from build123d import *

# Parameters (mm, degrees)
SKETCH_1_W          = 25
SKETCH_1_H          = 25
EXTRUDE_1_DEPTH     = 8
SKETCH_2_R          = 1.25
CUT_EXTRUDE_1_DEPTH = 50
SKETCH_3_R          = 1.25
CUT_EXTRUDE_2_DEPTH = 50
CUT_EXTRUDE_4_DEPTH = 10


with BuildPart() as part:
    # Эскиз1 → Бобышка-Вытянуть1 (new body)
    with BuildSketch(Plane.XY):
        Rectangle(SKETCH_1_W, SKETCH_1_H)
    extrude(amount=EXTRUDE_1_DEPTH)

    # Эскиз2 → Вырез-Вытянуть1 (cut)
    with BuildSketch(Plane(origin=(0, 12.5, 0), x_dir=(1, 0, 0), z_dir=(0, 1, 0))):
        with Locations(Location((-7.5, -4, 0), (0, 0, 270))):
            Circle(SKETCH_2_R)
        with Locations(Location((2.5, -4, 0), (0, 0, 270))):
            Circle(SKETCH_2_R)
    extrude(amount=-CUT_EXTRUDE_1_DEPTH, mode=Mode.SUBTRACT)

    # Эскиз3 → Вырез-Вытянуть2 (cut)
    with BuildSketch(Plane(origin=(12.5, 0, 0), x_dir=(0, 0, -1), z_dir=(1, 0, 0))):
        with Locations(Location((-4, 2.5, 0), (0, 0, 90))):
            Circle(SKETCH_3_R)
        with Locations(Location((-4, -7.5, 0), (0, 0, 90))):
            Circle(SKETCH_3_R)
    extrude(amount=-CUT_EXTRUDE_2_DEPTH, mode=Mode.SUBTRACT)

    # Эскиз4 → Вырез-Вытянуть4 (cut)
    with BuildSketch(Plane(origin=(0, 0, 0), x_dir=(-1, 0, 0), z_dir=(0, 0, -1))):
        Polygon((12.5, 7.5), (-7.5, -12.5), (12.5, -12.5), align=None)
    extrude(amount=-CUT_EXTRUDE_4_DEPTH, mode=Mode.SUBTRACT)


solid = part.part
Can you work these out from the model? Positions are in its coordinate system, mm. Give positions to 0.01 mm unless a question says otherwise; leave off trailing zeros. Loops run counter-clockwise (first coordinate to the right, second up) from the corner with the lowest first, then second, coordinate; pieces in that order, holes last. Notation, with made-up numbers: (-17.5, 30) - (-2.5, 30) arc R14 ccw to (-2.5, 43) - close; hole circle Ø11 at (55, 58.5). An arc over 180 degrees is marked (long way). One line per item, written item: value.
(1) If we section it at B-B, the plane x = -4.5: List the corners of the cut face in (y, z) for me, plus the area to 3 significant figures.
Verdict:
outline: (-0.5, 0) - (12.5, 0) - (12.5, 8) - (-0.5, 8) - close; hole circle Ø2.5 at (2.5, 4)
area: 99.1 mm^2
(2) If we section it at C-C, the plane y = 6.5: List the corners of the cut face in (x, z) for me, plus the area to 3 significant figures.
Verdict:
outline: (-11.5, 0) - (12.5, 0) - (12.5, 8) - (-11.5, 8) - close; hole circle Ø2.5 at (-7.5, 4); hole circle Ø2.5 at (2.5, 4)
area: 182 mm^2
(3) If we section it at D-D, the plane x = 9: List the corners of the cut face in (y, z) for me.
Verdict:
outline: (-12.5, 0) - (12.5, 0) - (12.5, 8) - (-12.5, 8) - close; hole circle Ø2.5 at (-7.5, 4); hole circle Ø2.5 at (2.5, 4)
(4) I'm going to push flat-ended pins straight in: pin 1 (2 mm diameter, centred on x = -1, z = 4.5, fed in from -Y); pin 2 (1.5 mm diameter, centred on y = -3, z = 7, fed in from -X); pin 3 (3 mm diameter, centred on y = 2.5, z = 4, fed in from -X); pin 4 (2 mm diameter, centred on y = 2.5, z = 4, fed in from -X). Where does each tip first touch, or does it pass through?
Verdict:
pin 1: y = -5
pin 2: x = -2.75
pin 3: x = -9
pin 4: through
(5) If we section it at A-A, the plane z = 3.25: List the corners of the cut face in (x, y) for me.
Verdict:
outline: (-12.5, 7.5) - (-8.5, 3.5) - (-8.5, 12.5) - (-12.5, 12.5) - close; (-6.5, 1.5) - (1.5, -6.5) - (1.5, 1.5) - close; (-6.5, 3.5) - (1.5, 3.5) - (1.5, 12.5) - (-6.5, 12.5) - close; (3.5, -8.5) - (7.5, -12.5) - (12.5, -12.5) - (12.5, -8.5) - close; (3.5, -6.5) - (12.5, -6.5) - (12.5, 1.5) - (3.5, 1.5) - close; (3.5, 3.5) - (12.5, 3.5) - (12.5, 12.5) - (3.5, 12.5) - close
(6) If we mould it in two halves opening along X, with no side actions, what happens to faces 1 (the face through (0, 12.5, 4)), 2 (the face through (2.88, -2.43, 5.19)), 3 (the face through (-12.5, 10, 4))? For each: released by +X, released by -X, zero draft, split by the parting line, or undercut.
Verdict:
face 1: zero draft
face 2: undercut
face 3: released by -X
(7) I need wall thicknesses on line 1 along Z through (x, y) = (-7.5, 7.25); line 2 along Y through (x, z) = (10.5, 4); line 3 along X through (y, z) = (5.75, 3.5). Which ranges of each line are inside material? Lowest first, please.
Verdict:
line 1: 0 to 2.75, 5.25 to 8
line 2: -12.5 to -8.75, -6.25 to 1.25, 3.75 to 12.5
line 3: -10.75 to -8.65, -6.35 to 1.35, 3.65 to 12.5
